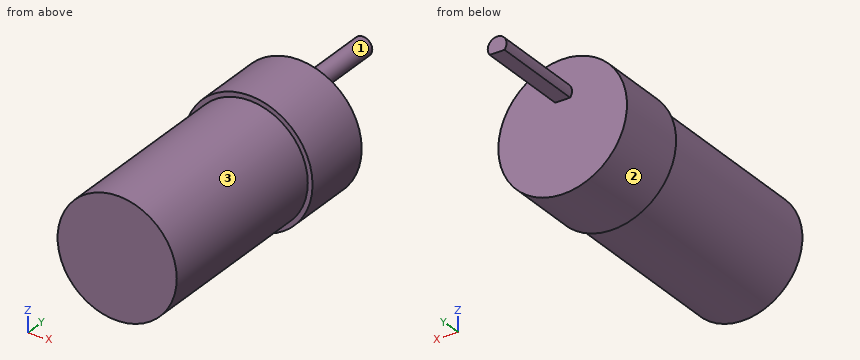
from build123d import *

# Parameters (mm, degrees)
F0_R     = 17.145
F1_DEPTH = 19.05
F3_DEPTH = 25.4
F4_R     = 15.875
F5_DEPTH = 50.8


with BuildPart() as f1:
    # F0 (on Front) → F1 (new body)
    with BuildSketch(Plane.XZ):
        Circle(F0_R)
    extrude(amount=F1_DEPTH)

    # F2 (on face) → F3 (join)
    with BuildSketch(Plane(origin=(0, 0, 0), x_dir=(-1, 0, 0), z_dir=(0, 1, 0))):
        with BuildLine():
            Line((-1.981773, 6.731), (1.981773, 6.731))
            ThreePointArc((1.981773, 6.731), (0, 10.755), (-1.981773, 6.731))
        make_face()
    extrude(amount=F3_DEPTH)

    # F4 (on face) → F5 (join)
    with BuildSketch(Plane.XZ.offset(19.05)):
        Circle(F4_R)
    extrude(amount=F5_DEPTH)


solid = f1.part
Input: part model. Units: mm. Frame: model coordinates. Face numbers are marked on the shaded views. A direction names the side the tool comes from. Give positions to 0.01 mm unless a question says otherwise; leave off trailing zeros. Order: outer loops, then holes, each group sorted by start corner. A loop starts at its lowest first (then second) coordinate and runs counter-clockwise, first axis right, second up. Notation, with made-up numbers: (86, -2.75) - (143, -2.75) arc R4 cw to (143, 2.25) - close; hole circle Ø1 at (-28, 28.5). An arc over 180 degrees is marked (long way). Answer as a JSON object with one key per item and string values. Group by question number.
Q1. Cut plane C-C, the plane y = -27. Output: boundary loops of the cut face in (x, z) (3 decimals), then the cut area to 3 significant figures.
Q2. Set-up query: the marked faces 1, 2 and 3. Return all of +Z, -Z, +X, -X, +Y, -Y with unobstructed straight access to the full face (end or side cutting, diameter ignored); none if empty.
Q3. Cut plane B-B, the plane z = 0. Output: boundary loops of the cut face in (x, y) (3 decimals), then the cut area to 3 significant figures.
Q4. First-contact query: pin 1 Ø4.5 at (x, y) = (-1, 10.5) entering from -Z; pin 2 Ø8 at (x, y) = (-9, -5) entering from +Z; pin 3 Ø12 at (x, y) = (8, -33) entering from -Z. Flat tips, straight axial feed; report the tip coordinate or a pass-through.
Q5. Cut plane A-A, the plane x = 0. Output: boundary loops of the cut face in (y, z) (3 decimals).
Q6. Line query: probe 1 along Y at (x, z) = (15, 0); probe 2 along X at (y, z) = (-52.5, -0.5); probe 3 along X at (y, z) = (-28.5, -5). Output: solid intervals per line, ascending.
Q7. Cut plane D-D, the plane x = -11.5. Output: boundary loops of the cut face in (y, z).
Results:
{
 "1": {"outline": "circle Ø31.75 at (0, 0)", "area": "792 mm^2"},
 "2": {"face 1": "+Y", "face 2": "+Y, -Y", "face 3": "-Y"},
 "3": {"outline": "(-17.145, -19.05) - (-15.875, -19.05) - (-15.875, -69.85) - (15.875, -69.85) - (15.875, -19.05) - (17.145, -19.05) - (17.145, 0) - (-17.145, 0) - close", "area": "2,270 mm^2"},
 "4": {"pin 1": "z = 6.73", "pin 2": "z = 16.4", "pin 3": "z = -15.75"},
 "5": {"outline": "(-69.85, -15.875) - (-19.05, -15.875) - (-19.05, -17.145) - (0, -17.145) - (0, 6.731) - (25.4, 6.731) - (25.4, 10.755) - (0, 10.755) - (0, 17.145) - (-19.05, 17.145) - (-19.05, 15.875) - (-69.85, 15.875) - close"},
 "6": {"probe 1": "-69.85 to 0", "probe 2": "-15.87 to 15.87", "probe 3": "-15.07 to 15.07"},
 "7": {"outline": "(-69.85, -10.94) - (-19.05, -10.94) - (-19.05, -12.72) - (0, -12.72) - (0, 12.72) - (-19.05, 12.72) - (-19.05, 10.94) - (-69.85, 10.94) - close"}
}
